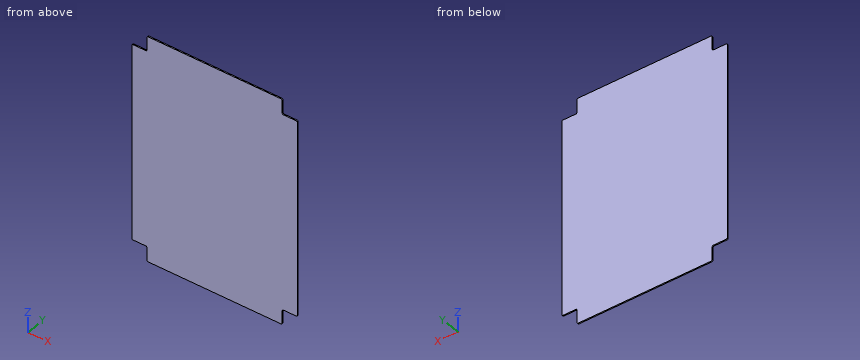
Autodesk Inventor part; units mm, degrees
ref_plane "YZ Plane" through (0, 0, 0) normal (1, 0, 0) x (0, 1, 0)
ref_plane "XZ Plane" through (0, 0, 0) normal (0, 1, 0) x (-1, 0, 0)
ref_plane "XY Plane" through (0, 0, 0) normal (0, 0, 1) x (1, 0, 0)
sketch "Sketch1" plane through (0, 0, 0) normal (0, 1, 0) x (-1, 0, 0)
  line L0 (186.6, -317.5) -> (-186.6, -317.5)
  line L1 (-228.6, -275.5) -> (-228.6, 275.5)
  line L2 (-186.6, 317.5) -> (186.6, 317.5)
  line L3 (228.6, 275.5) -> (228.6, -275.5)
  line L4 (186.6, -317.5) -> (186.6, -275.5)
  line L5 (186.6, -275.5) -> (228.6, -275.5)
  line L6 (-186.6, -317.5) -> (-186.6, -275.5)
  line L7 (-186.6, -275.5) -> (-228.6, -275.5)
  line L8 (186.6, 317.5) -> (186.6, 275.5)
  line L9 (186.6, 275.5) -> (228.6, 275.5)
  line L10 (-186.6, 317.5) -> (-186.6, 275.5)
  line L11 (-186.6, 275.5) -> (-228.6, 275.5)
  point P0 (0, 0)
  dimension "d5" = 457.2
  dimension "d6" = 228.6
  dimension "d7" = 635
  dimension "d8" = 317.5
  dimension "d9" = 42
extrude "Extrusion1" add sketch "Sketch1" along normal blind 3.175
fillet "Fillet1" radius 3.175 12 edges at (186.6, 1.5875, -317.5) (186.6, 1.5875, -275.5) (228.6, 1.5875, -275.5) (-186.6, 1.5875, -317.5) (-186.6, 1.5875, -275.5) (-228.6, 1.5875, -275.5) (-228.6, 1.5875, 275.5) (-186.6, 1.5875, 275.5) (-186.6, 1.5875, 317.5) (186.6, 1.5875, 317.5) (186.6, 1.5875, 275.5) (228.6, 1.5875, 275.5)
Part model, mm, in its own coordinate system. Round coordinates to 2 decimals unless told otherwise and drop trailing zeros. Order: outer loops, then holes, each group sorted by start corner. A loop starts at its lowest first (then second) coordinate and runs counter-clockwise, first axis right, second up. Notation, with made-up numbers: M 80,0 L 108,0 A17 cw 108,5 Z; hole C 85,56 d10. An arc over 180 degrees is marked long. Answer in a Markdown table with one row per item. Add a question column.
Q1. Pin check, flat tips, straight feed: pin 1 (1 mm diameter, centred on x = -202.5, y = 2, fed in from -Z); pin 2 (1.6 mm diameter, centred on y = 1, z = 290, fed in from -X); pin 3 (1.6 mm diameter, centred on y = 1.5, z = -288, fed in from +X). Stop position of each tip, or through.
Q2. Cut at A-A on y = 1.9. Give the cut face in (x, z) (3 decimals).
Q3. Wall check: L1, parallel to Z at x = 190.5, y = 0.6; L2, parallel to X at y = 1.8, z = -286.5. Give the ranges that are in metal, low to high. Write a range as from..to.
Q4. Cut at B-B on x = 198.5. Give the cut face in (y, z) (3 decimals), and give its area (3 significant figures).
Established:
| question | item | result |
|---|---|---|
| 1 | pin 1 | stops at z = -275.5 |
| 1 | pin 2 | stops at x = -186.6 |
| 1 | pin 3 | stops at x = 186.6 |
| 2 | outline | M -228.6,-272.325 A3.175 ccw -225.425,-275.5 L -189.775,-275.5 A3.175 cw -186.6,-278.675 L -186.6,-314.325 A3.175 ccw -183.425,-317.5 L 183.425,-317.5 A3.175 ccw 186.6,-314.325 L 186.6,-278.675 A3.175 cw 189.775,-275.5 L 225.425,-275.5 A3.175 ccw 228.6,-272.325 L 228.6,272.325 A3.175 ccw 225.425,275.5 L 189.775,275.5 A3.175 cw 186.6,278.675 L 186.6,314.325 A3.175 ccw 183.425,317.5 L -183.425,317.5 A3.175 ccw -186.6,314.325 L -186.6,278.675 A3.175 cw -189.775,275.5 L -225.425,275.5 A3.175 ccw -228.6,272.325 Z |
| 3 | L1 | z = -275.5..275.5 |
| 3 | L2 | x = -186.6..186.6 |
| 4 | outline | M 0,-275.5 L 3.175,-275.5 L 3.175,275.5 L 0,275.5 Z |
| 4 | area | 1,750 mm2 |
